Autodesk Inventor part; units mm, degrees
ref_plane "YZ Plane" through (0, 0, 0) normal (1, 0, 0) x (0, 1, 0)
ref_plane "XZ Plane" through (0, 0, 0) normal (0, 1, 0) x (-1, 0, 0)
ref_plane "XY Plane" through (0, 0, 0) normal (0, 0, 1) x (1, 0, 0)
sketch "Skizze1" plane through (0, 0, 0) normal (0, 0, 1) x (1, 0, 0)
  circle A0 centre (0, 0) radius 3.9
  dimension "d0" = 7.8
extrude "Extrusion1" add sketch "Skizze1" along normal blind 37
sketch "Skizze2" plane through (0, 0, 37) normal (0, 0, 1) x (1, 0, 0)
  circle A0 centre (0, 0) radius 5
  dimension "d3" = 10
extrude "Extrusion2" add sketch "Skizze2" along normal blind 1
chamfer "Fase1" distance 1 angle 45 1 edges at (-3.9, 0, 0)
properties part number "Bolzen" material "Edelstahl"
Work out the finished part from the listing and answer in its coordinate system (mm). A direction names the side the tool comes from. Give positions to 0.01 mm unless a question says otherwise; leave off trailing zeros. Loops run counter-clockwise (first coordinate to the right, second up) from the corner with the lowest first, then second, coordinate; pieces in that order, holes last. Notation, with made-up numbers: (49.5, -9.5) -> (66.5, -9.5) arc R16 ccw to (66.5, -0.5) -> close; hole circle Ø3 at (56, 41). An arc over 180 degrees is marked (long way). Put each result on its own line as item: value. Start each with the question number.
Item 1: Each of these flat-tipped pins is pushed along its axis until it touches: P1, Ø6, axis at x = -1, z = 16, coming from the +Y side; P2, Ø1, axis at y = 3.5, z = 32.5, coming from the +X side; P3, Ø1, axis at y = -1.5, z = 19, coming from the -X side. Where does it stop, or does it pass through?
Item 2: The part is cut by section D-D (y = 4.5). Give the vertices of the cut face in (x, z), then the cut area to 3 significant figures.
Item 3: The part is cut by section C-C (z = 32). Give the vertices of the cut face in (x, y).
Item 4: The part is cut by section A-A (y = 0). Give the vertices of the cut face in (x, z).
Item 5: Which of the six approach directions +Z, -Z, +X, -X, +Y, -Y give full straight-line access (tool end or side, diameter ignored) to faces 1 (the face through (0, 0, 38)), 2 (the face through (3, -3, 37))?
Item 6: Find the intervals of material crossed by L1, parallel to Z at x = 4.25, y = -1.5; L2, parallel to Y at x = 0, z = 33; L3, parallel to X at y = -2.75, z = 31, in increasing order. Write a range as [from, to].
Answers below:
1. P1: y = 3.9
1. P2: x = 2.49
1. P3: x = -3.77
2. outline: (-2.18, 37) -> (2.18, 37) -> (2.18, 38) -> (-2.18, 38) -> close
2. area: 4.36 mm2
3. outline: circle Ø7.8 at (0, 0)
4. outline: (-5, 37) -> (-3.9, 37) -> (-3.9, 1) -> (-2.9, 0) -> (2.9, 0) -> (3.9, 1) -> (3.9, 37) -> (5, 37) -> (5, 38) -> (-5, 38) -> close
5. face 1: +Z, +X, -X, +Y, -Y
5. face 2: -Z
6. L1: [37, 38]
6. L2: [-3.9, 3.9]
6. L3: [-2.77, 2.77]
